Model file for the job. Use its own axes, mm. A direction names the side the tool comes from. Round coordinates to 2 decimals unless told otherwise and drop trailing zeros. Order: outer loops, then holes, each group sorted by start corner. A loop starts at its lowest first (then second) coordinate and runs counter-clockwise, first axis right, second up. Notation, with made-up numbers: (4.25, 8) - (56.25, 8) arc R21 cw to (56.25, 30) - close; hole circle Ø8 at (87.5, 67.25). An arc over 180 degrees is marked (long way). Answer as CSV lines item,"result". Start each with the question number.
1. Band-saw the part on B-B on x = 70. List the corners of the cut face in (y, z) (3 decimals), then the cut area to 3 significant figures.
2. 3-axis set-ups, long thin cutter, end or side, ignore diameter. For faces 1 (the face through (6, 0, 3)), 2 (the face through (190.5, 56, 3)), 3 (the face through (38.1, -3, 3)), 4 (the face through (222, 0, 3)), 5 (the face through (107.95, 26, 3)): which of +Z, -Z, +X, -X, +Y, -Y reach the whole face in a straight line?
3. Pull direction Y, two halves, no side cores. Call faces 6 (the face through (113, 0, 3)), 7 (the face through (222, 52.72, 3)), 8 (the face through (170, 43.195, 3)): released by +Y, released by -Y, zero draft, split by the parting line, or undercut.
4. Band-saw the part on C-C on z = 2.75. State how many separate pieces and enclosed holes the cut face has, then the cut area to 3 significant figures.
5. Band-saw the part on D-D on x = 113.5. List the corners of the cut face in (y, z).
6. Band-saw the part on A-A on x = 25. List the corners of the cut face in (y, z), then the cut area to 3 significant figures.
7. Pin check, flat tips, straight feed: pin 1 Ø3 at (y, z) = (-2, 4) entering from +X; pin 2 Ø3 at (x, z) = (173.5, 4.5) entering from +Y; pin 3 Ø1.9 at (y, z) = (-1.5, 4) entering from -X. Stop position of each tip, or through.
8. Wall check: line 1 along Y through (x, z) = (170, 2.75) (3 decimals); line 2 along Y through (x, z) = (159.5, 5) (3 decimals); line 3 along X through (y, z) = (24.5, 5.5) (3 decimals). Give the ranges that are in metal, low to high. Write a range as [from, to].
```python
from build123d import *

# Parameters (mm, degrees)
BOSS_EXTRUDE1_DEPTH = 6.35
CUT_EXTRUDE1_DEPTH  = 237.19387672
FILLET1_R           = 2.54


with BuildPart() as part:
    # Sketch1 → Boss-Extrude1 (new body)
    with BuildSketch(Plane.XY):
        Polygon((0, 0), (12.7, 0), (12.7, -6.35), (38.1, -6.35), (38.1, 0), (190.5, 0), (190.5, -6.35), (215.9, -6.35), (215.9, 0), (228.6, 0), (228.6, 52.72), (215.9, 52.72), (215.9, 59.07), (190.5, 59.07), (190.5, 52.72), (38.1, 52.72), (38.1, 59.07), (12.7, 59.07), (12.7, 52.72), (0, 52.72), align=None)
    extrude(amount=BOSS_EXTRUDE1_DEPTH)

    # Sketch2 → Cut-Extrude1 (cut, through all)
    with BuildSketch(Plane.XY.offset(6.35)):
        Polygon((44.023573871, 26.36), (9.525, 38.161544143), (9.525, 14.558455857), align=None)
        Polygon((93.236073871, 43.195), (24.238926129, 43.195), (58.7375, 31.393455857), align=None)
        Polygon((107.95, 38.161544143), (73.451426129, 26.36), (107.95, 14.558455857), align=None)
        Polygon((93.236073871, 9.525), (58.7375, 21.326544143), (24.238926129, 9.525), align=None)
        Polygon((155.148573871, 26.36), (120.65, 38.161544143), (120.65, 14.558455857), align=None)
        Polygon((204.361073871, 43.195), (135.363926129, 43.195), (169.8625, 31.393455857), align=None)
        Polygon((219.075, 38.161544143), (184.576426129, 26.36), (219.075, 14.558455857), align=None)
        Polygon((204.361073871, 9.525), (169.8625, 21.326544143), (135.363926129, 9.525), align=None)
    extrude(amount=-CUT_EXTRUDE1_DEPTH, mode=Mode.SUBTRACT)

    # Fillet1
    fillet1_edges = [part.edges().sort_by_distance(p)[0] for p in [
        (73.451426129, 26.36, 3.175),
        (107.95, 38.161544143, 3.175),
        (107.95, 14.558455857, 3.175),
        (204.361073871, 9.525, 3.175),
        (135.363926129, 9.525, 3.175),
        (169.8625, 21.326544143, 3.175),
        (169.8625, 31.393455857, 3.175),
        (135.363926129, 43.195, 3.175),
        (204.361073871, 43.195, 3.175),
        (219.075, 14.558455857, 3.175),
        (184.576426129, 26.36, 3.175),
        (219.075, 38.161544143, 3.175),
        (9.525, 14.558455857, 3.175),
        (9.525, 38.161544143, 3.175),
        (44.023573871, 26.36, 3.175),
        (155.148573871, 26.36, 3.175),
        (120.65, 14.558455857, 3.175),
        (120.65, 38.161544143, 3.175),
        (24.238926129, 9.525, 3.175),
        (58.7375, 21.326544143, 3.175),
        (93.236073871, 9.525, 3.175),
        (58.7375, 31.393455857, 3.175),
        (24.238926129, 43.195, 3.175),
        (93.236073871, 43.195, 3.175),
    ]]
    fillet(fillet1_edges, radius=FILLET1_R)


solid = part.part
```
Reply:
1,outline,"(0, 0) - (9.525, 0) - (9.525, 6.35) - (0, 6.35) - close; (17.474, 0) - (35.246, 0) - (35.246, 6.35) - (17.474, 6.35) - close; (43.195, 0) - (52.72, 0) - (52.72, 6.35) - (43.195, 6.35) - close"
1,area,"234 mm2"
2,face 1,"+Z, -Z, -X, -Y"
2,face 2,"+Z, -Z, +Y"
2,face 3,"+Z, -Z, -Y"
2,face 4,"+Z, -Z, +X, -Y"
2,face 5,"+Z, -Z"
3,face 6,"released by -Y"
3,face 7,"released by +Y"
3,face 8,"undercut"
4,separate pieces,"1"
4,enclosed holes,"8"
4,area,"9,740 mm2"
5,outline,"(0, 0) - (52.72, 0) - (52.72, 6.35) - (0, 6.35) - close"
6,outline,"(-6.35, 0) - (19.85, 0) - (19.85, 6.35) - (-6.35, 6.35) - close; (32.87, 0) - (59.07, 0) - (59.07, 6.35) - (32.87, 6.35) - close"
6,area,"333 mm2"
7,pin 1,"stops at x = 215.9"
7,pin 2,"stops at y = 52.72"
7,pin 3,"stops at x = 12.7"
8,line 1,"y = [0, 9.525], [21.178, 31.542], [43.195, 52.72]"
8,line 2,"y = [0, 9.525], [17.782, 34.938], [43.195, 52.72]"
8,line 3,"x = [0, 9.525], [37.906, 79.569], [107.95, 120.65], [149.031, 190.694], [219.075, 228.6]"
